from build123d import *

# Parameters (mm, degrees)
SKETCH_1_W          = 20
SKETCH_1_H          = 20
EXTRUDE_1_DEPTH     = 10
SKETCH_1_3_W        = 5
SKETCH_1_3_H        = 10
SKETCH_1_3_W_2      = 10
EXTRUDE_2_DEPTH     = 20
SKETCH_2_W          = 5
SKETCH_2_H          = 5
CUT_EXTRUDE_1_DEPTH = 20
FILLET_1_R          = 10
SCALE_1_SCALE       = 0.2


with BuildPart() as part:
    # Sketch 1 → Extrude 1 (new body)
    with BuildSketch(Plane(origin=(0, 0, 0), x_dir=(1, 0, 0), z_dir=(0, 1, 0))):
        Rectangle(SKETCH_1_W, SKETCH_1_H)
        Polygon((-5, 5), (-5, -5), (5, 5), align=None, mode=Mode.SUBTRACT)
    extrude(amount=EXTRUDE_1_DEPTH)

    # Sketch 1_3 → Extrude 2 (add)
    with BuildSketch(Plane(origin=(0, 0, 0), x_dir=(1, 0, 0), z_dir=(0, 1, 0))):
        with Locations((-7.5, 15)):
            Rectangle(SKETCH_1_3_W, SKETCH_1_3_H)
        with Locations((0, 15)):
            Rectangle(SKETCH_1_3_W_2, SKETCH_1_3_H)
        with Locations((7.5, 15)):
            Rectangle(SKETCH_1_3_W, SKETCH_1_3_H)
    extrude(amount=EXTRUDE_2_DEPTH)

    # Sketch 2 → Cut-Extrude 1 (cut)
    with BuildSketch(Plane.XY.offset(-10)):
        Polygon((5, 20), (-5, 20), (5, 15), align=None)
        with Locations((7.5, 17.5)):
            Rectangle(SKETCH_2_W, SKETCH_2_H)
    extrude(amount=-CUT_EXTRUDE_1_DEPTH, mode=Mode.SUBTRACT)

    # Fillet 1
    fillet_1_edges = [part.edges().sort_by_distance(p)[0] for p in [
        (10, 5, 10),
    ]]
    fillet(fillet_1_edges, radius=FILLET_1_R)


with BuildPart() as part_1:
    # Scale 1: scaled about (-0.460547771, 6.995707008, -7.860015293)
    add(part.part.scale(SCALE_1_SCALE).moved(Location((-0.368438217, 5.596565606, -6.288012234))))


solid = part_1.part
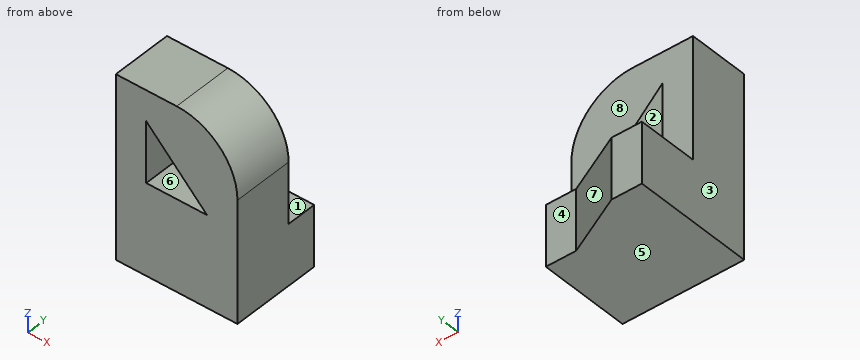
Geometry check sheet. Reference: the model listing, model coordinates, mm. Face numbers are marked on the shaded views. A direction names the side the tool comes from. Give positions to 0.01 mm unless a question says otherwise; leave off trailing zeros. Order: outer loops, then holes, each group sorted by start corner. A loop starts at its lowest first (then second) coordinate and runs counter-clockwise, first axis right, second up. Notation, with made-up numbers: (77.5, 35.25) - (90.5, 35.25) arc R25 ccw to (90.5, 58.25) - close; hole circle Ø2 at (64, -39). An arc over 180 degrees is marked (long way). Use one line per item in the form item = value.
1) Sectioned sample at A-A (z = -5.65). Record the boundary of the cut face in (x, y), and give its area (3 significant figures).
Working result:
outline = (-2.37, 5.6) - (-1.37, 5.6) - (-1.37, 7.6) - (-2.37, 7.6) - close; (-1.01, 5.6) - (1.53, 5.6) - (1.53, 7.6) - (-1.01, 7.6) - close
area = 7.07 mm^2
2) Depth check by flat-ended pin: pin 1 Ø0.6 at (x, y) = (-1, 9) entering from +Z; pin 2 Ø1.2 at (x, z) = (0, -6) entering from +Y. Enter the tip coordinate at first touch or a pass-through.
Working result:
pin_1 = -8.29
pin_2 = 7.6
3) Sectioned sample at B-B (x = -0.5). Record the boundary of the cut face in (y, z).
Working result:
outline = (5.6, -10.29) - (9.16, -10.29) - (9.16, -8.29) - (7.6, -8.29) - (7.6, -7.29) - (5.6, -7.29) - close; (5.6, -6.16) - (7.6, -6.16) - (7.6, -4.29) - (5.6, -4.29) - close
4) Sectioned sample at D-D (z = -9.65). Record the boundary of the cut face in (x, y), and give its area (3 significant figures).
Working result:
outline = (-2.37, 5.6) - (1.63, 5.6) - (1.63, 8.6) - (0.63, 8.6) - (-1.37, 9.6) - (-2.37, 9.6) - close
area = 14.0 mm^2
5) Sectioned sample at C-C (y = 6.15). Record the boundary of the cut face in (x, z), and give its area (3 significant figures).
Working result:
outline = (-2.37, -10.29) - (1.63, -10.29) - (1.63, -6.29) arc R2 ccw to (-0.37, -4.29) - (-2.37, -4.29) - close; hole (-1.37, -7.29) - (0.63, -7.29) - (-1.37, -5.29) - close
area = 21.1 mm^2
6) Draft check along X on the marked faces 6, 7 and 8. Enter one of: released by +X, released by -X, zero draft, split by the parting line, or undercut.
Working result:
face_6 = undercut
face_7 = released by +X
face_8 = zero draft
7) Access from +Z, -Z, +X, -X, +Y, -Y to the whole of each face (thin tool, end or side, straight path). Record for the marked faces 1, 2, 3, 4 and 5.
Working result:
face_1 = +Z, +X, -X, +Y
face_2 = +Y, -Y
face_3 = +Z, -Z, -X, +Y, -Y
face_4 = +Z, -Z, +X, +Y
face_5 = -Z, +X, -X, +Y, -Y
8) Material ranges on probe 1 along Y at (x, z) = (-1.7, -6.15); probe 2 along Y at (x, z) = (1.1, -8.9); probe 3 along Z at (x, y) = (-2.2, 8.5), recorded low to high. Write a range as from..to.
Working result:
probe_1 = 5.6..7.6
probe_2 = 5.6..8.6
probe_3 = -10.29..-8.29
